Geometry check sheet. Reference: the model listing, model coordinates, mm. A direction names the side the tool comes from. Coordinates: 2 decimals unless noted, no trailing zeros. Write each loop counter-clockwise with the first axis right and the second up, starting at its lowest first coordinate (ties: lowest second). Pieces come first, ordered by that corner, then holes. Notation, with made-up numbers: (36.5, 27.5) -> (60.5, 27.5) arc R7 ccw to (60.5, 38.5) -> close; hole circle Ø8 at (48, 62.5). An arc over 180 degrees is marked (long way). Answer in a Markdown table with one row per item. Add a question column.
Q1. Section check B-B, the plane z = 96.5. Record the boundary of the cut face in (x, y).
Q2. Gauge pin test, flat ends, axial feed: P1, Ø6.5, axis at x = 10, z = 270, coming from the +Y side; P2, Ø2.5, axis at x = 10, z = 50, coming from the +Y side (3 decimals). Record the tip position at first contact, or that the pin passes through.
Q3. Section check A-A, the plane y = 13.5. Record the boundary of the cut face in (x, z), and give its area (3 significant figures).
Q4. Tool access check on faces 4 (the face through (10, 2, 148)), 5 (the face through (10, 20, 148)). Record the directions out of +Z, -Z, +X, -X, +Y, -Y that give a thin tool (end or side, any length) a straight path to the whole face; none if there is none.
Q5. Thickness scan on line 1 (Y direction, x = 3.5, z = 65.5); line 2 (X direction, y = 0.5, z = 290). Record the ranges inside material, lowest first.
Q6. Release check for a two-part mould opening along Y. For faces 1 (the face through (10, 0, 148)), 2 (the face through (2, 10, 148)), 3 (the face through (1, 10, 300)) record: pulls with the +Y half, pulls with the -Y half, needs draft (parallel to the pull), parting line crosses it, or undercut.
```python
from build123d import *

# Parameters (mm, degrees)
SKETCH_1_W          = 20
SKETCH_1_H          = 20
SKETCH_1_W_2        = 16
SKETCH_1_H_2        = 16
EXTRUDE_1_DEPTH     = 300
SKETCH_2_R          = 2
CUT_EXTRUDE_1_DEPTH = 302.330383466


with BuildPart() as part:
    # 草图1 → 拉伸-薄壁1 (new body)
    with BuildSketch(Plane.XY):
        with Locations((10, 10)):
            Rectangle(SKETCH_1_W, SKETCH_1_H)
        with Locations((10, 10)):
            Rectangle(SKETCH_1_W_2, SKETCH_1_H_2, mode=Mode.SUBTRACT)
    extrude(amount=EXTRUDE_1_DEPTH)

    # 草图2 → 切除-拉伸1 (cut, through all)
    with BuildSketch(Plane(origin=(0, 20, 0), x_dir=(1, 0, 0), z_dir=(0, 1, 0))):
        with Locations(Location((10, -290, 0), (0, 0, 270))):
            Circle(SKETCH_2_R)
        with Locations(Location((10, -270, 0), (0, 0, 270))):
            Circle(SKETCH_2_R)
        with Locations(Location((10, -250, 0), (0, 0, 270))):
            Circle(SKETCH_2_R)
        with Locations(Location((10, -10, 0), (0, 0, 90))):
            Circle(SKETCH_2_R)
        with Locations(Location((10, -30, 0), (0, 0, 90))):
            Circle(SKETCH_2_R)
        with Locations(Location((10, -50, 0), (0, 0, 90))):
            Circle(SKETCH_2_R)
    extrude(amount=-CUT_EXTRUDE_1_DEPTH, mode=Mode.SUBTRACT)


solid = part.part
```
Calculated:
| question | item | result |
|---|---|---|
| 1 | outline | (0, 0) -> (20, 0) -> (20, 20) -> (0, 20) -> close; hole (2, 2) -> (18, 2) -> (18, 18) -> (2, 18) -> close |
| 2 | P1 | stops at y = 20 |
| 2 | P2 | passes through |
| 3 | outline | (0, 0) -> (2, 0) -> (2, 300) -> (0, 300) -> close; (18, 0) -> (20, 0) -> (20, 300) -> (18, 300) -> close |
| 3 | area | 1,200 mm² |
| 4 | face 4 | +Z, -Z |
| 4 | face 5 | +Z, -Z, +X, -X, +Y |
| 5 | line 1 | y = 0 to 2, 18 to 20 |
| 5 | line 2 | x = 0 to 8, 12 to 20 |
| 6 | face 1 | pulls with the -Y half |
| 6 | face 2 | undercut |
| 6 | face 3 | needs draft |
